```python
from build123d import *

# Parameters (mm, degrees)
SKETCH_R        = 4
PAD_DEPTH       = 744
POCKET_DEPTH    = 741
SKETCH001_R     = 15
SKETCH001_R_2   = 4
PAD001_DEPTH    = 745
SKETCH003_R     = 16
POCKET001_DEPTH = 1
SKETCH004_W     = 48
SKETCH004_H     = 15
POCKET002_DEPTH = 741


with BuildPart() as part:
    # Sketch → Pad (new body, symmetric)
    with BuildSketch(Plane.YZ):
        Polygon((23, 0), (49, 0), (56, 10), (67, 10), (69, 17), (72, 19), (72, 77), (59, 84), (13, 84), (0, 77), (0, 19), (3, 17), (5, 10), (16, 10), align=None)
        with Locations((36, 48)):
            Circle(SKETCH_R, mode=Mode.SUBTRACT)
        with BuildLine():
            ThreePointArc((27.5, 10), (25, 7.5), (27.5, 5))
            Line((27.5, 5), (44.5, 5))
            ThreePointArc((44.5, 5), (47, 7.5), (44.5, 10))
            Line((27.5, 10), (44.5, 10))
        make_face(mode=Mode.SUBTRACT)
    extrude(amount=PAD_DEPTH, both=True)

    # Sketch002 → Pocket (cut, symmetric)
    with BuildSketch(Plane.YZ):
        Polygon((11, 87.44), (17.5, 80.5), (54.5, 80.5), (61, 87.44), align=None)
    extrude(amount=POCKET_DEPTH, both=True, mode=Mode.SUBTRACT)

    # Sketch001 → Pad001 (join, symmetric)
    with BuildSketch(Plane(origin=(0, 0, 0), x_dir=(0, 1, 0), z_dir=(-1, 0, 0))):
        with Locations((36, -48)):
            Circle(SKETCH001_R)
        with Locations((36, -48)):
            Circle(SKETCH001_R_2, mode=Mode.SUBTRACT)
    extrude(amount=PAD001_DEPTH, both=True)

    # Sketch003 (on Face29 of Pad001) → Pocket001 (cut)
    with BuildSketch(Plane.XY.offset(80.5)):
        with Locations((-715, 36)):
            Circle(SKETCH003_R)
        with Locations((-660, 36)):
            Circle(SKETCH003_R)
        with Locations((-605, 36)):
            Circle(SKETCH003_R)
        with Locations((-550, 36)):
            Circle(SKETCH003_R)
        with Locations((-495, 36)):
            Circle(SKETCH003_R)
        with Locations((-440, 36)):
            Circle(SKETCH003_R)
        with Locations((-385, 36)):
            Circle(SKETCH003_R)
        with Locations((-330, 36)):
            Circle(SKETCH003_R)
        with Locations((-275, 36)):
            Circle(SKETCH003_R)
        with Locations((-220, 36)):
            Circle(SKETCH003_R)
        with Locations((-165, 36)):
            Circle(SKETCH003_R)
        with Locations((-110, 36)):
            Circle(SKETCH003_R)
        with Locations((-55, 36)):
            Circle(SKETCH003_R)
        with Locations((0, 36)):
            Circle(SKETCH003_R)
        with Locations((55, 36)):
            Circle(SKETCH003_R)
        with Locations((110, 36)):
            Circle(SKETCH003_R)
        with Locations((165, 36)):
            Circle(SKETCH003_R)
        with Locations((220, 36)):
            Circle(SKETCH003_R)
        with Locations((275, 36)):
            Circle(SKETCH003_R)
        with Locations((330, 36)):
            Circle(SKETCH003_R)
        with Locations((385, 36)):
            Circle(SKETCH003_R)
        with Locations((440, 36)):
            Circle(SKETCH003_R)
        with Locations((495, 36)):
            Circle(SKETCH003_R)
        with Locations((550, 36)):
            Circle(SKETCH003_R)
        with Locations((605, 36)):
            Circle(SKETCH003_R)
        with Locations((660, 36)):
            Circle(SKETCH003_R)
        with Locations((715, 36)):
            Circle(SKETCH003_R)
    extrude(amount=-POCKET001_DEPTH, mode=Mode.SUBTRACT)

    # Sketch004 → Pocket002 (cut, symmetric)
    with BuildSketch(Plane.YZ):
        with Locations((36, 7.5)):
            Rectangle(SKETCH004_W, SKETCH004_H)
    extrude(amount=POCKET002_DEPTH, both=True, mode=Mode.SUBTRACT)


solid = part.part
```
The listing builds one solid part. Answer for the finished solid, in the listing's coordinates (mm). A direction names the side the tool comes from. Coordinates: 2 decimals unless noted, no trailing zeros. Order: outer loops, then holes, each group sorted by start corner. A loop starts at its lowest first (then second) coordinate and runs counter-clockwise, first axis right, second up. Notation, with made-up numbers: M 62,35.5 L 75,35.5 A13 ccw 75,45.5 Z; hole C 73.25,3 d10. An arc over 180 degrees is marked long. Answer as a JSON object with one key per item and string values. Group by question number.
1. Flat-ended cylindrical pins translate along their axes: P1, Ø2, axis at y = 37, z = 15.5, coming from the -X side; P2, Ø8, axis at x = -79.5, y = 49.5, coming from the +Z side; P3, Ø19, axis at x = -55, y = 36, coming from the -Z side; P4, Ø6, axis at y = 33.5, z = 50, coming from the +X side. Find the tip coordinate at first contact, or state that the pin passes through.
2. Section A-A on x = 275 is taken. Write down the section's boundary in (y, z), then the cut area to 3 significant figures.
3. A tool of negligible diameter and unlimited length cuts with its end or side. For faces 1 (the cylindrical face through (314.015, 36.703, 80.007)), 2 (the flat face through (10, 36, 15)), from which of +Z, -Z, +X, -X, +Y, -Y can it reach the whole face along a straight path? Write none if from no direction.
4. Straight lines are drawn through the part: line 1 (Y direction, x = 605, z = 79.8); line 2 (Y direction, x = -715, z = 79.85); line 3 (X direction, y = 52, z = 26). For each, find the intervals that lie inside material, in ascending order.
Values follow:
{
 "1": {"P1": "x = -744", "P2": "z = 80.5", "P3": "z = 15", "P4": "x = 745"},
 "2": {"outline": "M 0,19 L 3,17 L 5,10 L 12,10 L 12,15 L 60,15 L 60,10 L 67,10 L 69,17 L 72,19 L 72,77 L 59,84 L 57.78,84 L 54.5,80.5 L 52,80.5 L 52,79.5 L 20,79.5 L 20,80.5 L 17.5,80.5 L 14.22,84 L 13,84 L 0,77 Z; hole C 36,48 d8", "area": "4,710 mm2"},
 "3": {"face 1": "+Z", "face 2": "-Z"},
 "4": {"line 1": "5.2 to 20, 52 to 66.8", "line 2": "5.29 to 20, 52 to 66.71", "line 3": "-744 to 744"}
}
